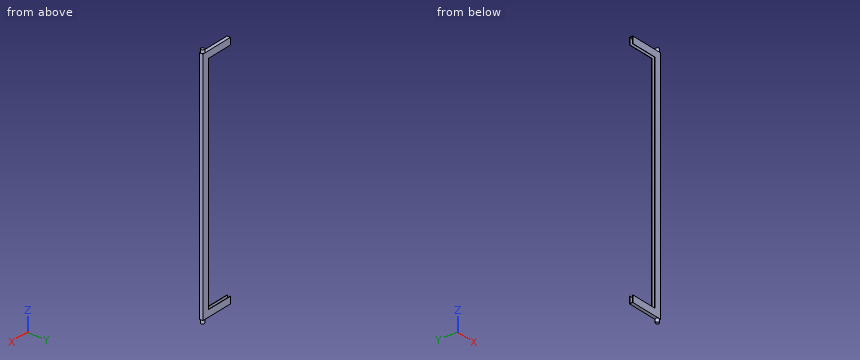
from build123d import *

# Parameters (mm, degrees)
CROQUIS1_W              = 100
CROQUIS1_H              = 700
SALIENTE_EXTRUIR1_DEPTH = 10
CROQUIS2_R              = 5
SALIENTE_EXTRUIR2_DEPTH = 10
SALIENTE_EXTRUIR3_START = 10
CROQUIS3_R              = 5
SALIENTE_EXTRUIR3_DEPTH = 10
CROQUIS4_W              = 698
CROQUIS4_H              = 8
CORTAR_EXTRUIR1_DEPTH   = 90
CROQUIS5_W              = 80
CROQUIS5_H              = 660
CORTAR_EXTRUIR2_DEPTH   = 10


with BuildPart() as part:
    # Croquis1 → Saliente-Extruir1 (new body)
    with BuildSketch(Plane(origin=(0, 0, 0), x_dir=(1, 0, 0), z_dir=(0, 1, 0))):
        Rectangle(CROQUIS1_W, CROQUIS1_H)
    extrude(amount=SALIENTE_EXTRUIR1_DEPTH)

    # Croquis2 → Saliente-Extruir2 (add)
    with BuildSketch(Plane.XY.offset(350)):
        with Locations((45, 5)):
            Circle(CROQUIS2_R)
    extrude(amount=SALIENTE_EXTRUIR2_DEPTH)

    # Croquis3 → Saliente-Extruir3 (add)
    with BuildSketch(Plane(origin=(0, 0, -350), x_dir=(-1, 0, 0), z_dir=(0, 0, -1)).offset(SALIENTE_EXTRUIR3_START)):
        with Locations(Location((-45, 5, 0), (0, 0, 180))):
            Circle(CROQUIS3_R)
    extrude(amount=-SALIENTE_EXTRUIR3_DEPTH)

    # Croquis4 → Cortar-Extruir1 (cut)
    with BuildSketch(Plane.ZY.offset(50)):
        with Locations((0, 5)):
            Rectangle(CROQUIS4_W, CROQUIS4_H)
    extrude(amount=-CORTAR_EXTRUIR1_DEPTH, mode=Mode.SUBTRACT)

    # Croquis5 → Cortar-Extruir2 (cut)
    with BuildSketch(Plane(origin=(0, 10, 0), x_dir=(1, 0, 0), z_dir=(0, 1, 0))):
        with Locations((-10, 0)):
            Rectangle(CROQUIS5_W, CROQUIS5_H)
    extrude(amount=-CORTAR_EXTRUIR2_DEPTH, mode=Mode.SUBTRACT)


solid = part.part
Geometry: final body of the model. Coordinates: model frame, mm. Coordinates: 2 decimals unless noted, no trailing zeros. Write each loop counter-clockwise with the first axis right and the second up, starting at its lowest first coordinate (ties: lowest second). Pieces come first, ordered by that corner, then holes. Notation, with made-up numbers: (64.5, -6) - (106.5, -6) arc R32 cw to (106.5, 26) - close; hole circle Ø2 at (31, 20.25). An arc over 180 degrees is marked (long way). Return JSON: item names as keys, results as strings.
Item 1: Section query C-C (y = 7.25). Output: boundary loops of the cut face in (x, z), and give its area (3 significant figures).
Completed:
{"outline": "(-50, -350) - (40.53, -350) - (40.53, -360) - (49.47, -360) - (49.47, -350) - (50, -350) - (50, 350) - (49.47, 350) - (49.47, 360) - (40.53, 360) - (40.53, 350) - (-50, 350) - (-50, 349) - (40, 349) - (40, -349) - (-50, -349) - close", "area": "7,360 mm2"}
Item 2: Section query A-A (x = -38.5). Output: boundary loops of the cut face in (y, z).
Completed:
{"outline": "(0, -350) - (10, -350) - (10, -330) - (9, -330) - (9, -349) - (1, -349) - (1, -330) - (0, -330) - close; (0, 330) - (1, 330) - (1, 349) - (9, 349) - (9, 330) - (10, 330) - (10, 350) - (0, 350) - close"}
Item 3: Pin query (flat end, axial travel): pin 1 Ø4 at (x, y) = (-30, 9) entering from +Z; pin 2 Ø0.5 at (x, y) = (0, 0.5) entering from -Z; pin 3 Ø0.8 at (y, z) = (0.5, 43) entering from -X. Return the tip coordinate at first contact, or that it passes through.
Completed:
{"pin 1": "stops at z = 350", "pin 2": "stops at z = -350", "pin 3": "stops at x = 30"}
Item 4: Line query: L1, parallel to Z at x = -2, y = 7.5; L2, parallel to Z at x = 2, y = 0.75; L3, parallel to X at y = 6, z = 223.5. Output: solid intervals per line, ascending.
Completed:
{"L1": "z = -350 to -349, 349 to 350", "L2": "z = -350 to -330, 330 to 350", "L3": "x = 40 to 50"}
Item 5: Section query B-B (z = 191.5). Output: boundary loops of the cut face in (x, y).
Completed:
{"outline": "(30, 0) - (50, 0) - (50, 10) - (30, 10) - (30, 9) - (40, 9) - (40, 1) - (30, 1) - close"}
